Could you check a few things on this model? Use its own coordinates, in mm. Coordinates: 2 decimals unless noted, no trailing zeros. Write each loop counter-clockwise with the first axis right and the second up, starting at its lowest first coordinate (ties: lowest second). Pieces come first, ordered by that corner, then holes. Notation, with made-up numbers: M 49.25,88.5 L 82.25,88.5 A13 ccw 82.25,95.5 Z; hole C 41.5,-22 d4. An arc over 180 degrees is marked long. Answer as CSV lines item,"result". Start each with the question number.
Item 1: Suppose I cut it at D-D, the plane y = -3. Write out the boundary of the cut face in (x, z).
Item 2: Suppose I cut it at B-B, the plane z = -15. Write out the boundary of the cut face in (x, y), and give its area (3 significant figures).
Item 3: Suppose I cut it at C-C, the plane x = 9. Write out the boundary of the cut face in (y, z).
Item 4: If I drill on line 1 along Y through (x, z) = (1.75, -0.25); line 2 along X through (y, z) = (-5.75, -15); line 3 along Y through (x, z) = (0.5, -0.75), over which ranges is the centre line in solid material (lowest first)? Write a range as [from, to].
Item 5: Suppose I cut it at A-A, the plane x = 5. Write out the boundary of the cut face in (y, z), and give its area (3 significant figures).
Item 6: I'm going to push flat-ended pins straight in: P1, Ø10, axis at y = 0, z = 0, coming from the +X side; P2, Ø4, axis at x = 3.5, y = 6.5, coming from the +Z side; P3, Ø6, axis at x = 5.5, z = 4, coming from the +Y side. Where does each tip first touch, or does it pass through?
Item 7: We'd pull the mould along Z, two halves only. Please class faces 1 (the flat face through (5, 9.5, -10)), 2 (the cylindrical face through (5.07, 0.13, -16.5)), 3 (the flat face through (5, 0, -20)): +Z half, -Z half, draft (parallel to the pull), parting line (faces both ways), or undercut.
```python
from build123d import *

# Parameters (mm, degrees)
SKETCH_1_R          = 5.462836395
EXTRUDE_1_DEPTH     = 10
SKETCH_2_R          = 1.5
CUT_EXTRUDE_1_DEPTH = 30.342801502


with BuildPart() as part:
    # 草图1 → 凸台-拉伸1 (new body)
    with BuildSketch(Plane(origin=(0, 0, 0), x_dir=(0, 0, -1), z_dir=(1, 0, 0))):
        with BuildLine():
            Line((0, 9.5), (20, 9.5))
            Line((20, 9.5), (20, -9.5))
            Line((20, -9.5), (0, -9.5))
            ThreePointArc((0, -9.5), (-6.717514421, -6.717514421), (-9.5, 0))
            ThreePointArc((-9.5, 0), (-6.717514421, 6.717514421), (0, 9.5))
        make_face()
        Circle(SKETCH_1_R, mode=Mode.SUBTRACT)
    extrude(amount=EXTRUDE_1_DEPTH)

    # 草图2 → 切除-拉伸1 (cut, through all)
    with BuildSketch(Plane(origin=(0, 9.5, 0), x_dir=(1, 0, 0), z_dir=(0, 1, 0))):
        with Locations(Location((5, 15, 0), (0, 0, 270))):
            Circle(SKETCH_2_R)
    extrude(amount=-CUT_EXTRUDE_1_DEPTH, mode=Mode.SUBTRACT)


solid = part.part
```
Ans:
1,outline,"M 0,-20 L 10,-20 L 10,-4.57 L 0,-4.57 Z; M 0,4.57 L 10,4.57 L 10,9.01 L 0,9.01 Z; hole C 5,-15 d3"
2,outline,"M 0,-9.5 L 3.5,-9.5 L 3.5,9.5 L 0,9.5 Z; M 6.5,-9.5 L 10,-9.5 L 10,9.5 L 6.5,9.5 Z"
2,area,"133 mm^2"
3,outline,"M -9.5,-20 L 9.5,-20 L 9.5,0 A9.5 ccw -9.5,0 Z; hole C 0,0 d10.93"
4,line 1,"y = [-9.5, -5.46], [5.46, 9.5]"
4,line 2,"x = [0, 3.5], [6.5, 10]"
4,line 3,"y = [-9.5, -5.41], [5.41, 9.5]"
5,outline,"M -9.5,-20 L 9.5,-20 L 9.5,-16.5 L -9.5,-16.5 Z; M -9.5,-13.5 L 9.5,-13.5 L 9.5,0 A9.5 ccw -9.5,0 Z; hole C 0,0 d10.93"
5,area,"371 mm^2"
6,P1,"passes through"
6,P2,"stops at z = 8.37"
6,P3,"stops at y = 9.45"
7,face 1,"draft"
7,face 2,"undercut"
7,face 3,"-Z half"
